Check sheet for the modelled part. Datum: model origin and axes. Units: mm. A direction names the side the tool comes from. Round coordinates to 2 decimals unless told otherwise and drop trailing zeros. Loops run counter-clockwise (first coordinate to the right, second up) from the corner with the lowest first, then second, coordinate; pieces in that order, holes last. Notation, with made-up numbers: (-0.5, 85.5) -> (40.5, 85.5) arc R28 ccw to (40.5, 112.5) -> close; hole circle Ø1 at (-17, -22.75). An arc over 180 degrees is marked (long way). Return JSON: item names as keys, results as strings.
from build123d import *

# Parameters (mm, degrees)
SKETCH1_W           = 20.5
SKETCH1_H           = 15
SKETCH1_R           = 1.5
BOSS_EXTRUDE1_DEPTH = 1.2
SKETCH2_W           = 1
SKETCH2_H           = 1
BOSS_EXTRUDE2_DEPTH = 8
SKETCH3_W           = 20.15
SKETCH3_H           = 2
BOSS_EXTRUDE3_DEPTH = 2


with BuildPart() as part:
    # Sketch1 → Boss-Extrude1 (new body)
    with BuildSketch(Plane(origin=(0, 0, 0), x_dir=(1, 0, 0), z_dir=(0, 1, 0))):
        Rectangle(SKETCH1_W, SKETCH1_H)
        with Locations(Location((-8.25, -5.5, 0), (0, 0, 270))):
            Circle(SKETCH1_R, mode=Mode.SUBTRACT)
        with Locations(Location((8.25, -5.5, 0), (0, 0, 90))):
            Circle(SKETCH1_R, mode=Mode.SUBTRACT)
    extrude(amount=BOSS_EXTRUDE1_DEPTH)

    # Sketch2 → Boss-Extrude2 (add)
    with BuildSketch(Plane(origin=(0, 0, 0), x_dir=(1, 0, 0), z_dir=(0, 1, 0))):
        with Locations((9.075, 6.4)):
            Rectangle(SKETCH2_W, SKETCH2_H)
        with Locations((6.4825, 6.4)):
            Rectangle(SKETCH2_W, SKETCH2_H)
        with Locations((3.89, 6.4)):
            Rectangle(SKETCH2_W, SKETCH2_H)
        with Locations((1.2975, 6.4)):
            Rectangle(SKETCH2_W, SKETCH2_H)
        with Locations((-1.295, 6.4)):
            Rectangle(SKETCH2_W, SKETCH2_H)
        with Locations((-3.8875, 6.4)):
            Rectangle(SKETCH2_W, SKETCH2_H)
        with Locations((-6.48, 6.4)):
            Rectangle(SKETCH2_W, SKETCH2_H)
        with Locations((-9.0725, 6.4)):
            Rectangle(SKETCH2_W, SKETCH2_H)
    extrude(amount=-BOSS_EXTRUDE2_DEPTH)

    # Sketch3 → Boss-Extrude3 (add)
    with BuildSketch(Plane(origin=(0, 0, 0), x_dir=(1, 0, 0), z_dir=(0, 1, 0))):
        with Locations((0, 6.4)):
            Rectangle(SKETCH3_W, SKETCH3_H)
    extrude(amount=-BOSS_EXTRUDE3_DEPTH)


solid = part.part
Q1. Material ranges on line 1 (X direction, y = 0.65, z = 5.5); line 2 (Z direction, x = 8.25, y = 0.75); line 3 (Y direction, x = 2, z = 7), recorded low to high.
Results list:
{"line 1": "-10.25 to -9.75, -6.75 to 6.75, 9.75 to 10.25", "line 2": "-7.5 to 4, 7 to 7.5", "line 3": "0 to 1.2"}
Q2. Draft check along X on faces 1 (the flat face through (4, -5, -5.9)), 2 (the flat face through (5.982, -5, -6.4)). Enter one of: released by +X, released by -X, zero draft, split by the parting line, or undercut.
Results list:
{"face 1": "zero draft", "face 2": "undercut"}
Q3. Go/stop test with flat-tipped pins: pin 1 (1.1 mm diameter, centred on x = 9, y = -5.5, fed in from +Z); pin 2 (4 mm diameter, centred on x = -3, y = -3.5, fed in from -Z); pin 3 (0.5 mm diameter, centred on x = -6.5, y = -4, fed in from -Z). Record where each tip stops, or that it passes through.
Results list:
{"pin 1": "z = -5.9", "pin 2": "z = -7.4", "pin 3": "z = -6.9"}
Q4. Section check A-A (z = 5.5). Record the boundary of the cut face in (x, y), then the cut area to 3 significant figures.
Results list:
{"outline": "(-10.25, 0) -> (-9.75, 0) -> (-9.75, 1.2) -> (-10.25, 1.2) -> close; (-6.75, 0) -> (6.75, 0) -> (6.75, 1.2) -> (-6.75, 1.2) -> close; (9.75, 0) -> (10.25, 0) -> (10.25, 1.2) -> (9.75, 1.2) -> close", "area": "17.4 mm^2"}
Q5. Section check C-C (y = -4.5). Count the separate pieces of the cut face and the enclosed holes in it, then the cut area to 3 significant figures.
Results list:
{"separate pieces": "8", "enclosed holes": "0", "area": "8.00 mm^2"}
Q6. Section check B-B (x = -8.25). Record the boundary of the cut face in (y, z).
Results list:
{"outline": "(-2, -7.4) -> (0, -7.4) -> (0, -7.5) -> (1.2, -7.5) -> (1.2, 4) -> (0, 4) -> (0, -5.4) -> (-2, -5.4) -> close; (0, 7) -> (1.2, 7) -> (1.2, 7.5) -> (0, 7.5) -> close"}
Q7. Tool access check on faces 3 (the flat face through (0, -1, -5.4)), 4 (the flat face through (6.5, -5, -6.9)), 5 (the flat face through (-4.388, -5, -6.4)). Record the directions out of +Z, -Z, +X, -X, +Y, -Y that give a thin tool (end or side, any length) a straight path to the whole face; none if there is none.
Results list:
{"face 3": "+Z, +X, -X, -Y", "face 4": "-Z, +X, -X, -Y", "face 5": "+Z, -Z, -Y"}
Q8. Section check D-D (y = -1.5). Record the boundary of the cut face in (x, z) (3 decimals), then the cut area to 3 significant figures.
Results list:
{"outline": "(-10.075, -7.4) -> (10.075, -7.4) -> (10.075, -5.4) -> (-10.075, -5.4) -> close", "area": "40.3 mm^2"}
